Part model, mm, in its own coordinate system. A direction names the side the tool comes from. Round coordinates to 2 decimals unless told otherwise and drop trailing zeros. Order: outer loops, then holes, each group sorted by start corner. A loop starts at its lowest first (then second) coordinate and runs counter-clockwise, first axis right, second up. Notation, with made-up numbers: M 47,28.5 L 53,28.5 A19 ccw 53,45.5 Z; hole C -26.5,51 d10. An arc over 180 degrees is marked long. Write each question's results on one line, items separated by ' | '. Start each with the question number.
1. Band-saw the part on C-C, the plane x = -23. List the corners of the cut face in (y, z).
2. Band-saw the part on A-A, the plane y = 16. List the corners of the cut face in (x, z).
3. Band-saw the part on D-D, the plane x = 2.5. List the corners of the cut face in (y, z), then the cut area to 3 significant figures.
4. Two-plate mould, pull along X, no slides. Class faces 6 (the face through (10.713, 7, 5)), 7 (the face through (-47.287, 7, 5)), 8 (the face through (-52.576, -16.501, 2.18)): +X half, -X half, draft (parallel to the pull), parting line (faces both ways), or undercut.
5. Band-saw the part on B-B, the plane z = 2.75. Give the number of separate pieces and of enclosed holes in the cut face, then the cut area to 3 significant figures.
6. Probe L1, parallel to X at y = 39.5, z = 2.5; L2, parallel to X at y = -28.5, z = 3.5; L3, parallel to X at y = -4.5, z = 4.5. List the from-to ranges inside material, lowest first. Write a range as [from, to].
7. Which spindle directions (+Z, -Z, +X, -X, +Y, -Y) get a long thin tool onto all of the face, cutting with end or side? Do faces 1 (the face through (15, -30.184, 3)), 2 (the face through (-47.287, 29, 2)), 3 (the face through (-30.787, 44, 3)), 4 (the face through (-51, 19.816, 3)), 5 (the face through (15, 19.816, 3)). Say none if no direction does.
8. Drop flat-ended pins along their axis: pin 1 Ø10 at (y, z) = (-30, 17.5) entering from +X; pin 2 Ø2 at (y, z) = (8.5, 6.5) entering from +X; pin 3 Ø1.5 at (x, y) = (-40.5, -51) entering from -Z; pin 4 Ø11 at (x, y) = (-18.29, -27.18) entering from -Z. Give the stop position or say it passes through.
```python
from build123d import *

# Parameters (mm, degrees)
CROQUIS2_R              = 22.5
CROQUIS2_W              = 8
CROQUIS2_H              = 25
CROQUIS2_W_2            = 25
CROQUIS2_H_2            = 8
SALIENTE_EXTRUIR1_DEPTH = 7
CROQUIS2_4_R            = 11.1
CROQUIS2_4_R_2          = 9
SALIENTE_EXTRUIR2_DEPTH = 22
CROQUIS2_5_R            = 22.5
CROQUIS2_5_R_2          = 11.1
SALIENTE_EXTRUIR3_DEPTH = 27
CROQUIS3_R              = 1.75
CORTAR_EXTRUIR1_DEPTH   = 7
CROQUIS4_R              = 3.1
CORTAR_EXTRUIR2_DEPTH   = 2.7
CROQUIS5_R              = 9
CROQUIS5_W              = 16.5
CROQUIS5_H              = 19.389278413
CORTAR_EXTRUIR3_DEPTH   = 4


with BuildPart() as part:
    # Croquis2 → Saliente-Extruir1 (new body)
    # profile 1 of 6: a face of its own
    with BuildSketch(Plane.XY):
        with BuildLine():
            Line((-5.786620614, -56.183989891), (3.713379386, -56.183989891))
            ThreePointArc((3.713379386, -56.183989891), (8.663126854, -54.133737359), (10.713379386, -49.183989891))
            Line((10.713379386, -49.183989891), (10.713379386, -30.183989891))
            Line((10.713379386, -30.183989891), (10.713379386, -5.183989891))
            Line((10.713379386, -5.183989891), (10.713379386, 19.816010109))
            Line((10.713379386, 19.816010109), (10.713379386, 39.205288522))
            Line((10.713379386, 39.205288522), (-5.786620614, 39.205288522))
            Line((-5.786620614, 39.205288522), (-30.786620614, 39.205288522))
            Line((-30.786620614, 39.205288522), (-47.286620614, 39.205288522))
            Line((-47.286620614, 39.205288522), (-47.286620614, 19.816010109))
            Line((-47.286620614, 19.816010109), (-47.286620614, -5.183989891))
            Line((-47.286620614, -5.183989891), (-47.286620614, -30.183989891))
            Line((-47.286620614, -30.183989891), (-47.286620614, -49.183989891))
            ThreePointArc((-47.286620614, -49.183989891), (-45.236368082, -54.133737359), (-40.286620614, -56.183989891))
            Line((-40.286620614, -56.183989891), (-30.786620614, -56.183989891))
            Line((-30.786620614, -56.183989891), (-5.786620614, -56.183989891))
        make_face()
        with Locations((-18.286620614, -27.183989891)):
            Circle(CROQUIS2_R, mode=Mode.SUBTRACT)
        with BuildLine():
            ThreePointArc((-29.286620614, 14.705288522), (-18.286620614, 3.705288522), (-7.286620614, 14.705288522))
            Line((-7.286620614, 14.705288522), (-7.286620614, 21.705288522))
            ThreePointArc((-7.286620614, 21.705288522), (-18.286620614, 32.705288522), (-29.286620614, 21.705288522))
            Line((-29.286620614, 21.705288522), (-29.286620614, 14.705288522))
        make_face(mode=Mode.SUBTRACT)
    # profile 2 of 6: a face of its own
    with BuildSketch(Plane.XY):
        Polygon((10.713379386, 39.205288522), (-5.786620614, 39.205288522), (-5.786620614, 48.816010109), (18.713379386, 48.816010109), (18.713379386, 19.816010109), (10.713379386, 19.816010109), align=None)
    # profile 3 of 6: a face of its own
    with BuildSketch(Plane.XY):
        Polygon((-47.286620614, 19.816010109), (-47.286620614, 39.205288522), (-30.786620614, 39.205288522), (-30.786620614, 48.816010109), (-55.286620614, 48.816010109), (-55.286620614, 19.816010109), align=None)
    # profile 4 of 6: a face of its own
    with BuildSketch(Plane.XY):
        with Locations((-51.286620614, -17.683989891)):
            Rectangle(CROQUIS2_W, CROQUIS2_H)
    # profile 5 of 6: a face of its own
    with BuildSketch(Plane.XY):
        with Locations((-18.286620614, -60.183989891)):
            Rectangle(CROQUIS2_W_2, CROQUIS2_H_2)
    # profile 6 of 6: a face of its own
    with BuildSketch(Plane.XY):
        with Locations((14.713379386, -17.683989891)):
            Rectangle(CROQUIS2_W, CROQUIS2_H)
    extrude(amount=SALIENTE_EXTRUIR1_DEPTH)



with BuildPart() as body_2:
    # Croquis2_4 → Saliente-Extruir2 (new body)
    with BuildSketch(Plane.XY):
        with Locations((-18.286620614, -27.183989891)):
            Circle(CROQUIS2_4_R)
        with Locations((-18.286620614, -27.183989891)):
            Circle(CROQUIS2_4_R_2, mode=Mode.SUBTRACT)
    extrude(amount=SALIENTE_EXTRUIR2_DEPTH)


with BuildPart() as part_1:
    add(part.part)

    add(body_2.part)  # Saliente-Extruir3 merges body 2
    # Croquis2_5 → Saliente-Extruir3 (add)
    with BuildSketch(Plane.XY):
        with Locations((-18.286620614, -27.183989891)):
            Circle(CROQUIS2_5_R)
        with Locations((-18.286620614, -27.183989891)):
            Circle(CROQUIS2_5_R_2, mode=Mode.SUBTRACT)
    extrude(amount=SALIENTE_EXTRUIR3_DEPTH)

    # Croquis3 → Cortar-Extruir1 (cut)
    with BuildSketch(Plane.XY.offset(7)):
        with Locations((-51.286620614, 34.316010109)):
            Circle(CROQUIS3_R)
        with Locations((-51.286620614, -17.683989891)):
            Circle(CROQUIS3_R)
        with Locations((-18.286620614, -60.183989891)):
            Circle(CROQUIS3_R)
        with Locations(Location((14.713379386, -17.683989891, 0), (0, 0, 180))):
            Circle(CROQUIS3_R)
        with Locations(Location((14.713379386, 34.316010109, 0), (0, 0, 180))):
            Circle(CROQUIS3_R)
    extrude(amount=-CORTAR_EXTRUIR1_DEPTH, mode=Mode.SUBTRACT)

    # Croquis4 → Cortar-Extruir2 (cut)
    with BuildSketch(Plane.XY.offset(7)):
        with Locations((-51.286620614, -17.683989891)):
            Circle(CROQUIS4_R)
        with Locations((-51.286620614, 34.316010109)):
            Circle(CROQUIS4_R)
        with Locations((14.713379386, 34.316010109)):
            Circle(CROQUIS4_R)
        with Locations((14.713379386, -17.683989891)):
            Circle(CROQUIS4_R)
        with Locations((-18.286620614, -60.183989891)):
            Circle(CROQUIS4_R)
    extrude(amount=-CORTAR_EXTRUIR2_DEPTH, mode=Mode.SUBTRACT)

    # Croquis5 → Cortar-Extruir3 (cut)
    # profile 1 of 4: a face of its own
    with BuildSketch(Plane(origin=(0, 0, 0), x_dir=(-1, 0, 0), z_dir=(0, 0, -1))):
        Polygon((30.786620614, 19.816010109), (30.786620614, 39.205288522), (5.786620614, 39.205288522), (5.786620614, 19.816010109), (-10.713379386, 19.816010109), (-10.713379386, -5.183989891), (-10.713379386, -30.183989891), (-10.713379386, -49.183989891), (47.286620614, -49.183989891), (47.286620614, -30.183989891), (47.286620614, -5.183989891), (47.286620614, 19.816010109), align=None)
        with Locations((18.286620614, -27.183989891)):
            Circle(CROQUIS5_R, mode=Mode.SUBTRACT)
        with BuildLine():
            Line((29.286620614, 21.705288522), (29.286620614, 14.705288522))
            ThreePointArc((29.286620614, 14.705288522), (18.286620614, 3.705288522), (7.286620614, 14.705288522))
            Line((7.286620614, 14.705288522), (7.286620614, 21.705288522))
            ThreePointArc((7.286620614, 21.705288522), (18.286620614, 32.705288522), (29.286620614, 21.705288522))
        make_face(mode=Mode.SUBTRACT)
    # profile 2 of 4: a face of its own
    with BuildSketch(Plane(origin=(0, 0, 0), x_dir=(-1, 0, 0), z_dir=(0, 0, -1))):
        with Locations((-2.463379386, 29.510649316)):
            Rectangle(CROQUIS5_W, CROQUIS5_H)
    # profile 3 of 4: a face of its own
    with BuildSketch(Plane(origin=(0, 0, 0), x_dir=(-1, 0, 0), z_dir=(0, 0, -1))):
        with Locations((39.036620614, 29.510649316)):
            Rectangle(CROQUIS5_W, CROQUIS5_H)
    # profile 4 of 4: a face of its own
    with BuildSketch(Plane(origin=(0, 0, 0), x_dir=(-1, 0, 0), z_dir=(0, 0, -1))):
        with BuildLine():
            ThreePointArc((40.286620614, -56.183989891), (45.236368082, -54.133737359), (47.286620614, -49.183989891))
            Line((47.286620614, -49.183989891), (-10.713379386, -49.183989891))
            ThreePointArc((-10.713379386, -49.183989891), (-8.663126854, -54.133737359), (-3.713379386, -56.183989891))
            Line((-3.713379386, -56.183989891), (5.786620614, -56.183989891))
            Line((5.786620614, -56.183989891), (30.786620614, -56.183989891))
            Line((30.786620614, -56.183989891), (40.286620614, -56.183989891))
        make_face()
    extrude(amount=-CORTAR_EXTRUIR3_DEPTH, mode=Mode.SUBTRACT)


solid = part_1.part
```
Solution:
1) outline: M -64.18,0 L -56.18,0 L -56.18,4 L -34.85,4 L -34.85,22 L -37.23,22 L -37.23,27 L -49.18,27 L -49.18,7 L -64.18,7 Z; M -19.52,4 L 4.77,4 L 4.77,7 L -5.18,7 L -5.18,27 L -17.13,27 L -17.13,22 L -19.52,22 Z; M 31.64,4 L 39.21,4 L 39.21,7 L 31.64,7 Z
2) outline: M -47.29,4 L -29.29,4 L -29.29,7 L -47.29,7 Z; M -7.29,4 L 10.71,4 L 10.71,7 L -7.29,7 Z
3) outline: M -56.18,4 L 39.21,4 L 39.21,0 L 48.82,0 L 48.82,7 L -18.57,7 L -18.57,27 L -35.8,27 L -35.8,7 L -56.18,7 Z | area: 698 mm^2
4) face 6: +X half | face 7: -X half | face 8: undercut
5) separate pieces: 5 | enclosed holes: 5 | area: 1,330 mm^2
6) L1: [-55.29, -30.79], [-5.79, 18.71] | L2: [-55.29, -47.29], [10.71, 18.71] | L3: [-47.29, 10.71]
7) face 1: +Z, -Z, +X, -Y | face 2: -Z, -Y | face 3: +Z, -Z, +Y | face 4: +Z, -Z, -X | face 5: +Z, -Z, +X
8) pin 1: x = 4.21 | pin 2: x = 10.71 | pin 3: z = 4 | pin 4: through
